from build123d import *

# Parameters (mm, degrees)
SKETCH1_R           = 5.5
BOSS_EXTRUDE1_DEPTH = 13
SKETCH2_R           = 3
CUT_EXTRUDE1_DEPTH  = 7
CHAMFER1_SIZE       = 2.5
CHAMFER1_SIZE_2     = 5.361267301
SKETCH3_W           = 11.617421712
SKETCH3_H           = 2
CUT_EXTRUDE2_DEPTH  = 7
SKETCH4_R           = 2.5
CUT_EXTRUDE3_DEPTH  = 7
SKETCH5_R           = 1
CUT_EXTRUDE5_DEPTH  = 4


with BuildPart() as part:
    # Sketch1 → Boss-Extrude1 (new body)
    with BuildSketch(Plane(origin=(0, 0, 0), x_dir=(1, 0, 0), z_dir=(0, 1, 0))):
        with Locations(Location((0, 0, 0), (0, 0, 90))):
            Circle(SKETCH1_R)
    extrude(amount=BOSS_EXTRUDE1_DEPTH)

    # Sketch2 → Cut-Extrude1 (cut)
    with BuildSketch(Plane(origin=(0, 13, 0), x_dir=(1, 0, 0), z_dir=(0, 1, 0))):
        with Locations(Location((0, 0, 0), (0, 0, 270))):
            Circle(SKETCH2_R)
    extrude(amount=-CUT_EXTRUDE1_DEPTH, mode=Mode.SUBTRACT)

    # Chamfer1
    # the kernel refuses this chamfer: 5.361267301, 2.5 mm, written as the material it takes off along each edge
    with BuildSketch(Plane(origin=(0, 13, 0), x_dir=(0, 0, 1), z_dir=(-1, 0, 0))) as chamfer1_piece_1:
        Polygon((3 + CHAMFER1_SIZE, 0), (3, -CHAMFER1_SIZE_2), (3, 0), align=None)
    revolve(axis=Axis((0, 13, 0), (0, 1, 0)), mode=Mode.SUBTRACT)

    # Sketch3 → Cut-Extrude2 (cut)
    with BuildSketch(Plane(origin=(0, 13, 0), x_dir=(-1, 0, 0), z_dir=(0, -1, 0))):
        Rectangle(SKETCH3_W, SKETCH3_H)
    extrude(amount=CUT_EXTRUDE2_DEPTH, mode=Mode.SUBTRACT)

    # Sketch4 → Cut-Extrude3 (cut)
    with BuildSketch(Plane.XZ):
        with Locations(Location((0, 0, 0), (0, 0, 270))):
            Circle(SKETCH4_R)
    extrude(amount=-CUT_EXTRUDE3_DEPTH, mode=Mode.SUBTRACT)

    # Sketch5 → Cut-Extrude5 (cut)
    with BuildSketch(Plane(origin=(0, 0, -5.5), x_dir=(-1, 0, 0), z_dir=(0, 0, -1))):
        with Locations(Location((0, 4, 0), (0, 0, 90))):
            Circle(SKETCH5_R)
    extrude(amount=-CUT_EXTRUDE5_DEPTH, mode=Mode.SUBTRACT)


solid = part.part
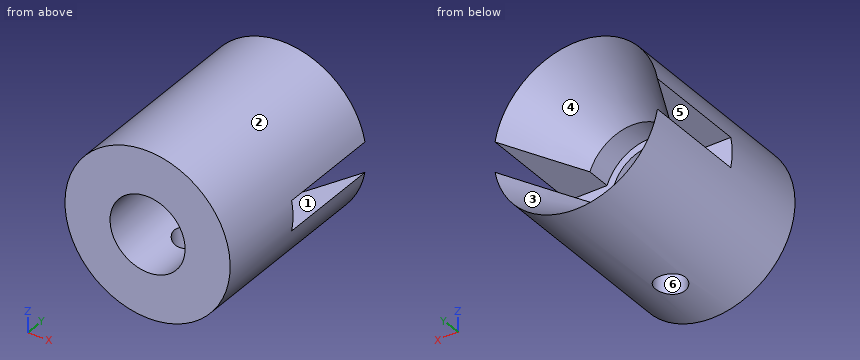
Verification items for the finished model (mm, model axes). Face numbers are marked on the shaded views. A direction names the side the tool comes from. Coordinates: 2 decimals unless noted, no trailing zeros. Order: outer loops, then holes, each group sorted by start corner. A loop starts at its lowest first (then second) coordinate and runs counter-clockwise, first axis right, second up. Notation, with made-up numbers: M 76.5,61.25 L 123.5,61.25 A32 cw 123.5,100.25 Z; hole C 46,-19.5 d10. An arc over 180 degrees is marked long. One line per item, written item: value. Start each with the question number.
Item 1: Sectioned sample at B-B on z = 0. Record the cut outline in (x, y).
Item 2: Depth check by flat-ended pin: P1, Ø1.5, axis at y = 7, z = 1, coming from the -X side; P2, Ø0.8, axis at x = -3.5, y = 10.5, coming from the +Z side; P3, Ø2, axis at x = -2.5, y = 3, coming from the +Z side. Enter the tip coordinate at first touch or a pass-through.
Item 3: Thickness scan on probe 1 along X at (y, z) = (2.5, 0); probe 2 along Y at (x, z) = (-2.75, 0.25); probe 3 along Z at (x, y) = (-1.75, 2.25). Record the ranges inside material, lowest first.
Item 4: Sectioned sample at A-A on x = 0. Record the cut outline in (y, z), then the cut area to 3 significant figures.
Item 5: Mould release check, pull along X, two halves, no side actions. Record for the marked faces 1, 2 and 3: pulls with the +X half, pulls with the -X half, needs draft (parallel to the pull), parting line crosses it, or undercut.
Item 6: Sectioned sample at D-D on y = 1.75. Record the cut outline in (x, z).
Item 7: Sectioned sample at C-C on y = 10.5. Record the cut outline in (x, z).
Item 8: Access from +Z, -Z, +X, -X, +Y, -Y to the whole of each face (thin tool, end or side, straight path). Record for the marked faces 4, 5 and 6.
Calculated:
1. outline: M -5.5,0 L -2.5,0 L -2.5,6 L -5.5,6 Z; M 2.5,0 L 5.5,0 L 5.5,6 L 2.5,6 Z
2. P1: x = -5.41
2. P2: z = 4.54
2. P3: z = 5.29
3. probe 1: -5.5 to -2.5, 2.5 to 5.5
3. probe 2: 0 to 6
3. probe 3: -5.21 to -1.79, 1.79 to 5.21
4. outline: M 0,-5.5 L 3,-5.5 L 3,-2.5 L 0,-2.5 Z; M 0,2.5 L 6,2.5 L 6,3 L 7.64,3 L 13,5.5 L 0,5.5 Z; M 5,-5.5 L 13,-5.5 L 7.64,-3 L 6,-3 L 6,-2.5 L 5,-2.5 Z
4. area: 51.6 mm^2
5. face 1: needs draft
5. face 2: parting line crosses it
5. face 3: undercut
6. outline: C 0,0 d11; hole C 0,0 d5
7. outline: M -5.41,-1 A5.5 ccw 5.41,-1 L 4.22,-1 A4.33 cw -4.22,-1 Z; M -5.41,1 L -4.22,1 A4.33 cw 4.22,1 L 5.41,1 A5.5 ccw Z
8. face 4: +Y
8. face 5: +X, -X, +Y
8. face 6: -Z
